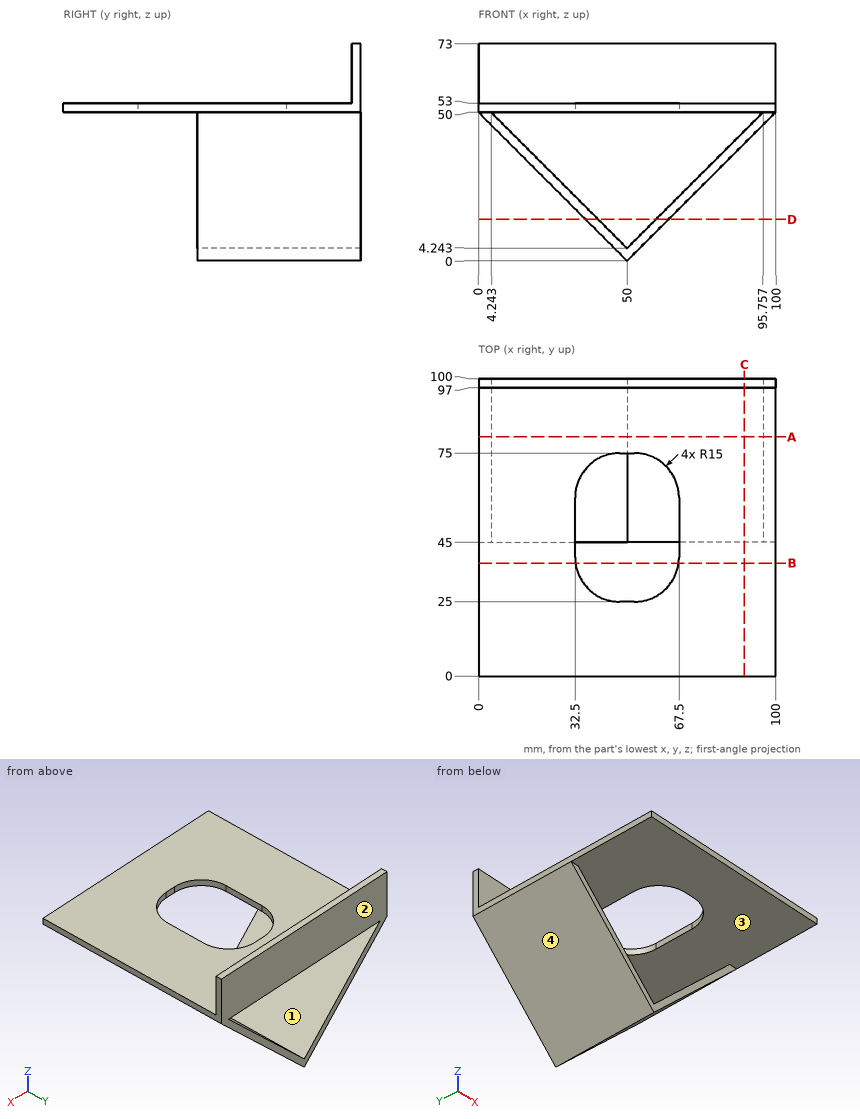
Design review of the part shown in the three views and the two pictorial views. Dimensions are in mm from the part's minimum x, y and z. Give positions to 0.01 mm unless a question says otherwise; leave off trailing zeros. Loops run counter-clockwise (first coordinate to the right, second up) from the corner with the lowest first, then second, coordinate; pieces in that order, holes last. Notation, with made-up numbers: (-16, 89) -> (9, 89) arc R30 cw to (9, 123) -> close; hole circle Ø9 at (81, 0.5). An arc over 180 degrees is marked (long way). One line per item, written item: value.
Q1. We need section C-C on x = 89.5. Give the boundary of the cut face in (y, z).
Numbers:
outline: (0, 50) -> (100, 50) -> (100, 73) -> (97, 73) -> (97, 53) -> (0, 53) -> close; (45, 39.5) -> (100, 39.5) -> (100, 43.74) -> (45, 43.74) -> close
Q2. We need section B-B on y = 38. Give the boundary of the cut face in (x, z), and give its area (3 significant figures).
Numbers:
outline: (0, 50) -> (32.63, 50) -> (32.63, 53) -> (0, 53) -> close; (67.37, 50) -> (100, 50) -> (100, 53) -> (67.37, 53) -> close
area: 196 mm^2
Q3. For pin 1 Ø4 at (y, z) = (83.5, 11.5) entering from +X; pin 2 Ø4 at (x, y) = (60.5, 79.5) entering from +Z; pin 3 Ø6 at (y, z) = (40, 22) entering from +X, all flat-tipped, find the tip position at first contact; note any pin that passes through.
Numbers:
pin 1: stops at x = 63.5
pin 2: stops at z = 53
pin 3: passes through
Q4. For L1, parallel to Y at x = 65, z = 66; L2, parallel to Z at x = 87, y = 23.5; L3, parallel to X at y = 64.5, z = 26.5 (1 decimal), list the stretches that pass through material, from the lowest coordinate up.
Numbers:
L1: y = 97 to 100
L2: z = 50 to 53
L3: x = 23.5 to 27.7, 72.3 to 76.5
Q5. We need section D-D on z = 14. Give the boundary of the cut face in (x, y).
Numbers:
outline: (36, 45) -> (40.24, 45) -> (40.24, 100) -> (36, 100) -> close; (59.76, 45) -> (64, 45) -> (64, 100) -> (59.76, 100) -> close
Q6. Draft analysis for pull direction X (two halves, no side actions). For the marked faces 1, 2, 3 and 4, state which applies: pulls with the +X half, pulls with the -X half, needs draft (parallel to the pull), parting line crosses it, or undercut.
Numbers:
face 1: undercut
face 2: needs draft
face 3: undercut
face 4: pulls with the -X half
Q7. We need section A-A on y = 80.5. Give the boundary of the cut face in (x, z).
Numbers:
outline: (0, 50) -> (50, 0) -> (100, 50) -> (100, 53) -> (0, 53) -> close; hole (4.24, 50) -> (50, 4.24) -> (95.76, 50) -> close
